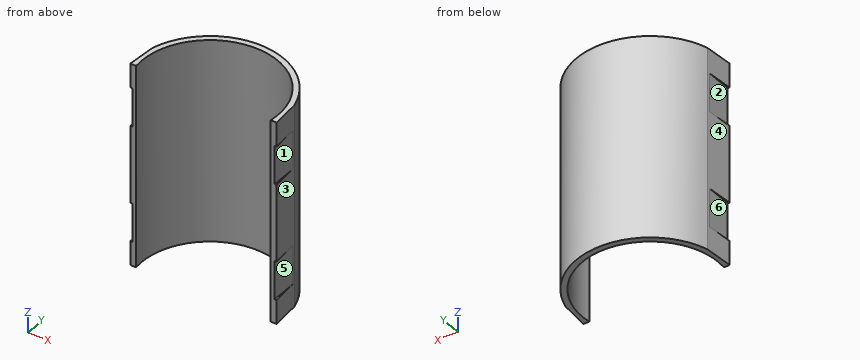
Autodesk Fusion 360 part; units mm, degrees
sketch "Sketch1" plane through (0, 0, 0) normal (0, 0, 1) x (1, 0, 0)
  line L0 (0, 0) -> (-70, 0)
  line L1 (-35, 0) -> (-35, 40)
  arc A0 (0, 0) -> (-70, 0) centre (-35, 4.6875) ccw
  line L2 (-70, 0) -> (-73, 0)
  line L3 (0, 0) -> (3, 0)
  line L4 (-35, 40) -> (-35, 43)
  arc A1 (3, 0) -> (-73, 0) centre (-35, 4.7093) ccw
  line L5 (-73, 0) -> (-71.8933, 14.9591)
  line L6 (3, 0) -> (1.8933, 14.9591)
  dimension "d1" = 70
  dimension "d2" = 40
  dimension "d3" = 3
  dimension "d4" = 3
  dimension "d5" = 3
  dimension "d6" = 15
  dimension "d7" = 15
extrude "Extrude1" add sketch "Sketch1" along normal blind 105 contours A0 L3 L4 A1 L6 | A0 L2 L4 A1 L5
sketch "Sketch4" plane through (0, 0, 0) normal (0, -1, 0) x (1, 0, 0)
  line L0 (-73, 0) -> (-70, 0)
  line L1 (-70, 0) -> (-70, 105)
  line L2 (-70, 105) -> (-73, 105)
  line L3 (-73, 105) -> (-73, 0)
  line L4 (-73, 105) -> (3, 105)
  line L5 (3, 105) -> (3, 0)
  line L6 (3, 0) -> (-73, 0)
  line L7 (-73, 0) -> (-73, 105)
  line L8 (-73, 52.5) -> (-73, 72.5)
  line L9 (-73, 72.5) -> (-73, 92.5)
  line L10 (-73, 92.5) -> (-72, 92.5)
  line L11 (-72, 92.5) -> (-72, 72.5)
  line L12 (-72, 72.5) -> (-73, 72.5)
  line L13 (-73, 72.5) -> (-73, 92.5)
  line L14 (-73, 52.5) -> (3, 52.5) construction
  line L15 (-35, 52.5) -> (-35, 93.5456) construction
  line L16 (-73, 32.5) -> (-73, 12.5)
  line L17 (-72, 12.5) -> (-72, 32.5)
  line L18 (-73, 12.5) -> (-72, 12.5)
  line L19 (-72, 32.5) -> (-73, 32.5)
  line L20 (3, 92.5) -> (2, 92.5)
  line L21 (2, 72.5) -> (3, 72.5)
  line L22 (3, 72.5) -> (3, 92.5)
  line L23 (2, 92.5) -> (2, 72.5)
  line L24 (3, 72.5) -> (3, 92.5)
  line L25 (2, 32.5) -> (3, 32.5)
  line L26 (3, 32.5) -> (3, 12.5)
  line L27 (2, 12.5) -> (2, 32.5)
  line L28 (3, 12.5) -> (2, 12.5)
  dimension "d31" = 20
  dimension "d32" = 20
  dimension "d33" = 1
  dimension "d34" = 76
extrude "Extrude6" cut sketch "Sketch4" against normal blind 20 contours L3 L7 L16 L17 L18 L19 | L5 L25 L26 L27 L28 | L3 L7 L9 L10 L11 L12 L13 | L5 L20 L21 L22 L23 L24
Check sheet for the modelled part. Datum: model origin and axes. Units: mm. Face numbers are marked on the shaded views. A direction names the side the tool comes from. Give positions to 0.01 mm unless a question says otherwise; leave off trailing zeros. Order: outer loops, then holes, each group sorted by start corner. A loop starts at its lowest first (then second) coordinate and runs counter-clockwise, first axis right, second up. Notation, with made-up numbers: (66.5, 41.5) -> (97.5, 41.5) arc R19 cw to (97.5, 76.5) -> close; hole circle Ø8 at (11, -7.5). An arc over 180 degrees is marked (long way). Return JSON: item names as keys, results as strings.
1. Cross-section at B-B, the plane z = 75. Record the cut outline in (x, y) (1 decimal), plus the area to 3 significant figures.
From the geometry:
{"outline": "(-72, 0) -> (-70, 0) arc R35.3 cw (long way) to (0, 0) -> (2, 0) -> (2, 13.5) -> (1.9, 15) arc R38.3 ccw to (-71.9, 15) -> (-72, 13.5) -> close", "area": "346 mm^2"}
2. Cross-section at D-D, the plane x = -35. Record the cut outline in (y, z), plus the area to 3 significant figures.
From the geometry:
{"outline": "(40, 0) -> (43, 0) -> (43, 105) -> (40, 105) -> close", "area": "315 mm^2"}
3. Set-up check for the marked faces 1, 2 and 3: record each of +Z, -Z, +X, -X, +Y, -Y from which the full face is reachable in a straight line by a thin tool's end or side.
From the geometry:
{"face 1": "+X, +Y, -Y", "face 2": "-X, +Y, -Y", "face 3": "+Z, -Z, +X, +Y"}
4. Material ranges on probe 1 along Y at (x, z) = (-35, 65); probe 2 along X at (y, z) = (24.5, 57.5); probe 3 along X at (y, z) = (24, 15), recorded low to high. Write a range as [from, to].
From the geometry:
{"probe 1": "[40, 43]", "probe 2": "[-67.78, -64.23], [-5.77, -2.22]", "probe 3": "[-68.08, -64.56], [-5.44, -1.92]"}
5. Mould release check, pull along Z, two halves, no side actions. Record for the marked faces 4, 5 and 6: +Z half, -Z half, draft (parallel to the pull), parting line (faces both ways), or undercut.
From the geometry:
{"face 4": "draft", "face 5": "undercut", "face 6": "undercut"}
6. Go/stop test with flat-tipped pins: P1, Ø15, axis at y = 8.5, z = 27.5, coming from the +X side; P2, Ø11, axis at y = 6.5, z = 82, coming from the +X side; P3, Ø1.5, axis at y = 28.5, z = 88, coming from the -X side. Record where each tip stops, or that it passes through.
From the geometry:
{"P1": "x = 2.78", "P2": "x = 2", "P3": "x = -65.58"}
7. Cross-section at A-A, the plane y = 7. Record the cut outline in (x, z).
From the geometry:
{"outline": "(-72.48, 0) -> (-70.24, 0) -> (-70.24, 105) -> (-72.48, 105) -> (-72.48, 92.5) -> (-72, 92.5) -> (-72, 72.5) -> (-72.48, 72.5) -> (-72.48, 32.5) -> (-72, 32.5) -> (-72, 12.5) -> (-72.48, 12.5) -> close; (0.24, 0) -> (2.48, 0) -> (2.48, 12.5) -> (2, 12.5) -> (2, 32.5) -> (2.48, 32.5) -> (2.48, 72.5) -> (2, 72.5) -> (2, 92.5) -> (2.48, 92.5) -> (2.48, 105) -> (0.24, 105) -> close"}
8. Cross-section at C-C, the plane y = 23. Record the cut outline in (x, z), plus the area to 3 significant figures.
From the geometry:
{"outline": "(-68.64, 0) -> (-65.19, 0) -> (-65.19, 105) -> (-68.64, 105) -> close; (-4.81, 0) -> (-1.36, 0) -> (-1.36, 105) -> (-4.81, 105) -> close", "area": "724 mm^2"}
